```python
from build123d import *

# Parameters (mm, degrees)
F0_W         = 1524
F0_H         = 2032
F0_R         = 88.6274236121
F1_DEPTH     = 254
F2_R         = 5.08
F3_T1_DEPTH  = 254
F3_T4_ANGLE  = 90
F3_T6_ANGLE  = 90
F3_T8_ANGLE  = 90
F3_T10_ANGLE = 90
F3_T12_ANGLE = 90
F3_T14_ANGLE = 90
F3_T16_ANGLE = 90
F3_T18_ANGLE = 90


# Not quite as in the source:
# - a fillet or chamfer that OpenCascade refuses, or shapes differently, is made with other operations: its cross-section is extruded or revolved along the edge and cut away or added


with BuildPart() as f1:
    # F0 (on Top) → F1 (new body)
    with BuildSketch(Plane.XY):
        Rectangle(F0_W, F0_H)
        with Locations((0, 860.7016801834)):
            Circle(F0_R, mode=Mode.SUBTRACT)
    extrude(amount=F1_DEPTH)

    # F2
    f2_edges = [f1.edges().sort_by_distance(p)[0] for p in [
        (-762, 0, 254),
        (0, -1016, 254),
        (762, 0, 254),
        (0, 1016, 254),
        (0, 1016, 0),
        (762, 0, 0),
        (0, -1016, 0),
        (-762, 0, 0),
    ]]
    fillet(f2_edges, radius=F2_R)

    # F3: fillet of radius 19.05 on 4 edges, made by hand

    # F3_s2 → F3_t1 (cut)
    with BuildSketch(Plane.XY):
        with BuildLine():
            ThreePointArc((762, 996.95), (756.4203841816, 1010.4203841816), (742.95, 1016))
            Line((742.95, 1016), (762, 1016))
            Line((762, 1016), (762, 996.95))
        make_face()
        with BuildLine():
            ThreePointArc((762, -996.95), (756.4203841816, -1010.4203841816), (742.95, -1016))
            Line((742.95, -1016), (762, -1016))
            Line((762, -1016), (762, -996.95))
        make_face()
        with BuildLine():
            ThreePointArc((-742.95, -1016), (-756.4203841816, -1010.4203841816), (-762, -996.95))
            Line((-762, -996.95), (-762, -1016))
            Line((-762, -1016), (-742.95, -1016))
        make_face()
        with BuildLine():
            ThreePointArc((-742.95, 1016), (-756.4203841816, 1010.4203841816), (-762, 996.95))
            Line((-762, 996.95), (-762, 1016))
            Line((-762, 1016), (-742.95, 1016))
        make_face()
    extrude(amount=F3_T1_DEPTH, mode=Mode.SUBTRACT)

    # F3_s3 → F3_t4 (revolve, cut)
    with BuildSketch(Plane.XZ.offset(-996.95)):
        with BuildLine():
            ThreePointArc((-756.92, 0), (-760.5121024484, 1.4878975516), (-762, 5.08))
            Line((-762, 5.08), (-762, 0))
            Line((-762, 0), (-756.92, 0))
        make_face()
    revolve(axis=Axis((-742.95, 996.95, 0), (0, 0, -1)), revolution_arc=F3_T4_ANGLE, mode=Mode.SUBTRACT)

    # F3_s5 → F3_t6 (revolve, cut)
    with BuildSketch(Plane.YZ.offset(-742.95)):
        with BuildLine():
            ThreePointArc((1010.92, 254), (1014.5121024484, 252.5121024484), (1016, 248.92))
            Line((1016, 248.92), (1016, 254))
            Line((1016, 254), (1010.92, 254))
        make_face()
    revolve(axis=Axis((-742.95, 996.95, 254), (0, 0, 1)), revolution_arc=F3_T6_ANGLE, mode=Mode.SUBTRACT)

    # F3_s7 → F3_t8 (revolve, cut)
    with BuildSketch(Plane.YZ.offset(-742.95)):
        with BuildLine():
            ThreePointArc((-1010.92, 0), (-1014.5121024484, 1.4878975516), (-1016, 5.08))
            Line((-1016, 5.08), (-1016, 0))
            Line((-1016, 0), (-1010.92, 0))
        make_face()
    revolve(axis=Axis((-742.95, -996.95, 0), (0, 0, -1)), revolution_arc=F3_T8_ANGLE, mode=Mode.SUBTRACT)

    # F3_s9 → F3_t10 (revolve, cut)
    with BuildSketch(Plane.XZ.offset(996.95)):
        with BuildLine():
            ThreePointArc((-756.92, 254), (-760.5121024484, 252.5121024484), (-762, 248.92))
            Line((-762, 248.92), (-762, 254))
            Line((-762, 254), (-756.92, 254))
        make_face()
    revolve(axis=Axis((-742.95, -996.95, 254), (0, 0, 1)), revolution_arc=F3_T10_ANGLE, mode=Mode.SUBTRACT)

    # F3_s11 → F3_t12 (revolve, cut)
    with BuildSketch(Plane.XZ.offset(996.95)):
        with BuildLine():
            ThreePointArc((756.92, 0), (760.5121024484, 1.4878975516), (762, 5.08))
            Line((762, 5.08), (762, 0))
            Line((762, 0), (756.92, 0))
        make_face()
    revolve(axis=Axis((742.95, -996.95, 0), (0, 0, -1)), revolution_arc=F3_T12_ANGLE, mode=Mode.SUBTRACT)

    # F3_s13 → F3_t14 (revolve, cut)
    with BuildSketch(Plane.YZ.offset(742.95)):
        with BuildLine():
            ThreePointArc((-1010.92, 254), (-1014.5121024484, 252.5121024484), (-1016, 248.92))
            Line((-1016, 248.92), (-1016, 254))
            Line((-1016, 254), (-1010.92, 254))
        make_face()
    revolve(axis=Axis((742.95, -996.95, 254), (0, 0, 1)), revolution_arc=F3_T14_ANGLE, mode=Mode.SUBTRACT)

    # F3_s15 → F3_t16 (revolve, cut)
    with BuildSketch(Plane.YZ.offset(742.95)):
        with BuildLine():
            ThreePointArc((1010.92, 0), (1014.5121024484, 1.4878975516), (1016, 5.08))
            Line((1016, 5.08), (1016, 0))
            Line((1016, 0), (1010.92, 0))
        make_face()
    revolve(axis=Axis((742.95, 996.95, 0), (0, 0, -1)), revolution_arc=F3_T16_ANGLE, mode=Mode.SUBTRACT)

    # F3_s17 → F3_t18 (revolve, cut)
    with BuildSketch(Plane.XZ.offset(-996.95)):
        with BuildLine():
            ThreePointArc((756.92, 254), (760.5121024484, 252.5121024484), (762, 248.92))
            Line((762, 248.92), (762, 254))
            Line((762, 254), (756.92, 254))
        make_face()
    revolve(axis=Axis((742.95, 996.95, 254), (0, 0, 1)), revolution_arc=F3_T18_ANGLE, mode=Mode.SUBTRACT)


solid = f1.part
```
Can you work these out from the model? Positions are in its coordinate system, mm. Coordinates: 2 decimals unless noted, no trailing zeros. Write each loop counter-clockwise with the first axis right and the second up, starting at its lowest first coordinate (ties: lowest second). Pieces come first, ordered by that corner, then holes. Notation, with made-up numbers: (2, 57.25) - (13, 57.25) arc R31 cw to (13, 88.25) - close; hole circle Ø2 at (67, -18). An arc over 180 degrees is marked (long way). Return JSON: item names as keys, results as strings.
Q1. Please list where these lines run through material, in increasing order: L1, parallel to Y at x = 0, z = 155.5; L2, parallel to Y at x = 24, z = 83.5; L3, parallel to X at y = 890, z = 73. Write a range as from..to.
Computed values:
{"L1": "y = -1016..772.07, 949.33..1016", "L2": "y = -1016..775.39, 946.02..1016", "L3": "x = -762..-83.64, 83.64..762"}
Q2. If we section it at B-B (y = 806.5): Please give me the cut outline in (x, z).
Computed values:
{"outline": "(-762, 5.08) arc R5.08 ccw to (-756.92, 0) - (-70.12, 0) - (-70.12, 254) - (-756.92, 254) arc R5.08 ccw to (-762, 248.92) - close; (70.12, 0) - (756.92, 0) arc R5.08 ccw to (762, 5.08) - (762, 248.92) arc R5.08 ccw to (756.92, 254) - (70.12, 254) - close"}
Q3. Thinking about a two-plate mould opening in X: for faces 1 (the flat face through (762, -14, 125)), 2 (the flat face through (-762, -14, 125)), 3 (the flat face through (-10, -1016, 125)), 4 (the cylindrical face through (-11.538, 948.575, 125.222)), which applies, +X half, -X half, draft (parallel to the pull), parting line (faces both ways), or undercut?
Computed values:
{"face 1": "+X half", "face 2": "-X half", "face 3": "draft", "face 4": "undercut"}
Q4. If we section it at A-A (x = 0): Please give me the cut outline in (y, z).
Computed values:
{"outline": "(-1016, 5.08) arc R5.08 ccw to (-1010.92, 0) - (772.07, 0) - (772.07, 254) - (-1010.92, 254) arc R5.08 ccw to (-1016, 248.92) - close; (949.33, 0) - (1010.92, 0) arc R5.08 ccw to (1016, 5.08) - (1016, 248.92) arc R5.08 ccw to (1010.92, 254) - (949.33, 254) - close"}
